The figure shows three views and two pictorial views of one solid part (mm, origin at its lowest corner). Answer the questions. A direction names the side the tool comes from. Round coordinates to 2 decimals unless told otherwise and drop trailing zeros. Write each loop counter-clockwise with the first axis right and the second up, starting at its lowest first coordinate (ties: lowest second). Pieces come first, ordered by that corner, then holes.
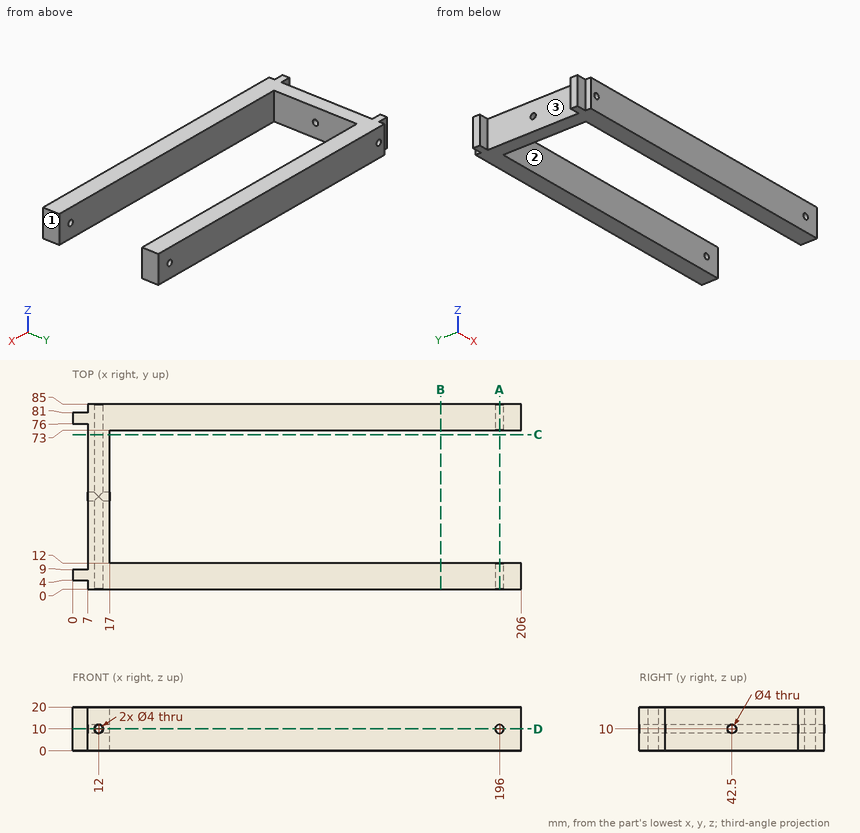
Q1. Straight lines are drawn through the part: probe 1 along Y at (x, z) = (47, 12.25); probe 2 along Z at (x, y) = (12, 32); probe 3 along X at (y, z) = (16.5, 10). For each, find the intervals that lie inside material, in ascending order.
Verdict:
probe 1: y = 0 to 12, 73 to 85
probe 2: z = 0 to 8, 12 to 20
probe 3: x = 7 to 10, 14 to 17
Q2. Which of the six approach directions +Z, -Z, +X, -X, +Y, -Y give full straight-line access (tool end or side, diameter ignored) to the marked faces 1, 2 and 3?
Verdict:
face 1: +Z, -Z, +X, +Y, -Y
face 2: +Z, -Z, +X
face 3: +Z, -Z, -X
Q3. Flat-ended cylindrical pins translate along their axes: pin 1 Ø5 at (x, z) = (196, 10) entering from -Y; pin 2 Ø3.5 at (x, z) = (2, 7.5) entering from +Y; pin 3 Ø4.5 at (y, z) = (42.5, 10) entering from -X; pin 4 Ø1 at (y, z) = (42, 4.5) entering from +X. Find the tip coordinate at first contact, or state that the pin passes through.
Verdict:
pin 1: stops at y = 0
pin 2: stops at y = 81
pin 3: stops at x = 7
pin 4: stops at x = 17
Q4. Section A-A (x = 196) is taken. Determine the outline of the cut face in (y, z), then the cut area to 3 significant figures.
Verdict:
outline: (0, 0) - (12, 0) - (12, 8) - (0, 8) - close; (0, 12) - (12, 12) - (12, 20) - (0, 20) - close; (73, 0) - (85, 0) - (85, 8) - (73, 8) - close; (73, 12) - (85, 12) - (85, 20) - (73, 20) - close
area: 384 mm2
Q5. Section C-C (y = 71) is taken. Determine the outline of the cut face in (x, z), then the cut area to 3 significant figures.
Verdict:
outline: (7, 0) - (17, 0) - (17, 20) - (7, 20) - close; hole circle Ø4 at (12, 10)
area: 187 mm2
Q6. Section B-B (x = 169) is taken. Determine the outline of the cut face in (y, z).
Verdict:
outline: (0, 0) - (12, 0) - (12, 20) - (0, 20) - close; (73, 0) - (85, 0) - (85, 20) - (73, 20) - close
Q7. Section D-D (z = 10) is taken. State how many separate pieces and enclosed holes the cut face has, then the cut area to 3 significant figures.
Verdict:
separate pieces: 6
enclosed holes: 0
area: 5,000 mm2
